from build123d import *

# Parameters (mm, degrees)
SKETCH_2_R          = 7
EXTRUDE_1_DEPTH     = 10
SKETCH_3_R          = 10.5
EXTRUDE_2_DEPTH     = 9
SKETCH_4_R          = 3.5
CUT_EXTRUDE_1_DEPTH = 25.114311104
CUT_EXTRUDE_START   = -13
SKETCH_5_R          = 5.5
CUT_EXTRUDE_2_DEPTH = 2.5


with BuildPart() as part:
    # Эскиз2 → Бобышка-Вытянуть1 (new body)
    with BuildSketch(Plane.XY):
        Circle(SKETCH_2_R)
    extrude(amount=EXTRUDE_1_DEPTH)

    # Эскиз3 → Бобышка-Вытянуть2 (add)
    with BuildSketch(Plane(origin=(0, 0, 0), x_dir=(-1, 0, 0), z_dir=(0, 0, -1))):
        Circle(SKETCH_3_R)
    extrude(amount=EXTRUDE_2_DEPTH)

    # Эскиз4 → Вырез-Вытянуть1 (cut, through all)
    with BuildSketch(Plane.XY.offset(10)):
        Circle(SKETCH_4_R)
    extrude(amount=-CUT_EXTRUDE_1_DEPTH, mode=Mode.SUBTRACT)

    # Эскиз5 → Вырез-Вытянуть2 (cut)
    with BuildSketch(Plane.XY.offset(10).offset(CUT_EXTRUDE_START)):
        Circle(SKETCH_5_R)
    extrude(amount=-CUT_EXTRUDE_2_DEPTH, mode=Mode.SUBTRACT)


solid = part.part
Geometry: final body of the model. Coordinates: model frame, mm. A direction names the side the tool comes from. Give positions to 0.01 mm unless a question says otherwise; leave off trailing zeros. Order: outer loops, then holes, each group sorted by start corner. A loop starts at its lowest first (then second) coordinate and runs counter-clockwise, first axis right, second up. Notation, with made-up numbers: (77, -31) -> (91, -31) arc R13 ccw to (91, -13) -> close; hole circle Ø5 at (-28.75, 64.25). An arc over 180 degrees is marked (long way). Put each result on its own line as item: value.
Q1. Section C-C, the plane z = -6.5. Return loops of the section in (x, y), then the cut area to 3 significant figures.
Here are the results:
outline: circle Ø21 at (0, 0); hole circle Ø7 at (0, 0)
area: 308 mm^2
Q2. Reachability of faces 4 (the face through (4, 0, -3)), 5 (the face through (-10, 3.2, -4.4)), 6 (the face through (-2, -7, 0)) from +Z, -Z, +X, -X, +Y, -Y: full face, straight path, thin tool, end or side. Return the list, or none.
Here are the results:
face 4: none
face 5: +Z, -Z
face 6: +Z
Q3. Section A-A, the plane y = 0. Return loops of the section in (x, z), then the cut area to 3 significant figures.
Here are the results:
outline: (-10.5, -9) -> (-3.5, -9) -> (-3.5, -5.5) -> (-5.5, -5.5) -> (-5.5, -3) -> (-3.5, -3) -> (-3.5, 10) -> (-7, 10) -> (-7, 0) -> (-10.5, 0) -> close; (3.5, -9) -> (10.5, -9) -> (10.5, 0) -> (7, 0) -> (7, 10) -> (3.5, 10) -> (3.5, -3) -> (5.5, -3) -> (5.5, -5.5) -> (3.5, -5.5) -> close
area: 186 mm^2
Q4. Pin query (flat end, axial travel): pin 1 (5 mm diameter, centred on y = -0.5, z = 5.5, fed in from -X); pin 2 (3 mm diameter, centred on y = 2.5, z = 3.5, fed in from +X); pin 3 (1.5 mm diameter, centred on y = -7, z = 4, fed in from -X). Return the tip coordinate at first contact, or that it passes through.
Here are the results:
pin 1: stops at x = -7
pin 2: stops at x = 6.93
pin 3: stops at x = -3.15
Q5. Section D-D, the plane z = 2.25. Return loops of the section in (x, y).
Here are the results:
outline: circle Ø14 at (0, 0); hole circle Ø7 at (0, 0)
Q6. Material intervals for L1, parallel to Y at x = 0, z = -4.2; L2, parallel to Y at x = 0, z = 5; L3, parallel to Z at x = 2, y = -3, sorted ascending.
Here are the results:
L1: y = -10.5 to -5.5, 5.5 to 10.5
L2: y = -7 to -3.5, 3.5 to 7
L3: z = -9 to -5.5, -3 to 10
Q7. Draft query along Z for faces 1 (the face through (-5, 0, -9)), 2 (the face through (3.233, -1.341, 3.591)), 3 (the face through (4, 0, -5.5)). Return one class per face: released by +Z, released by -Z, zero draft, split by the parting line, or undercut.
Here are the results:
face 1: released by -Z
face 2: zero draft
face 3: undercut
